Drawing for the job (mm, zero at the part's lowest x, y, z). A direction names the side the tool comes from. Give positions to 0.01 mm unless a question says otherwise; leave off trailing zeros. Loops run counter-clockwise (first coordinate to the right, second up) from the corner with the lowest first, then second, coordinate; pieces in that order, holes last. Notation, with made-up numbers: M 54,0 L 86,0 A4 ccw 86,4 Z; hole C -34.5,3 d5. An arc over 180 degrees is marked long. Answer in a Markdown table with one row per item. Add a question column.
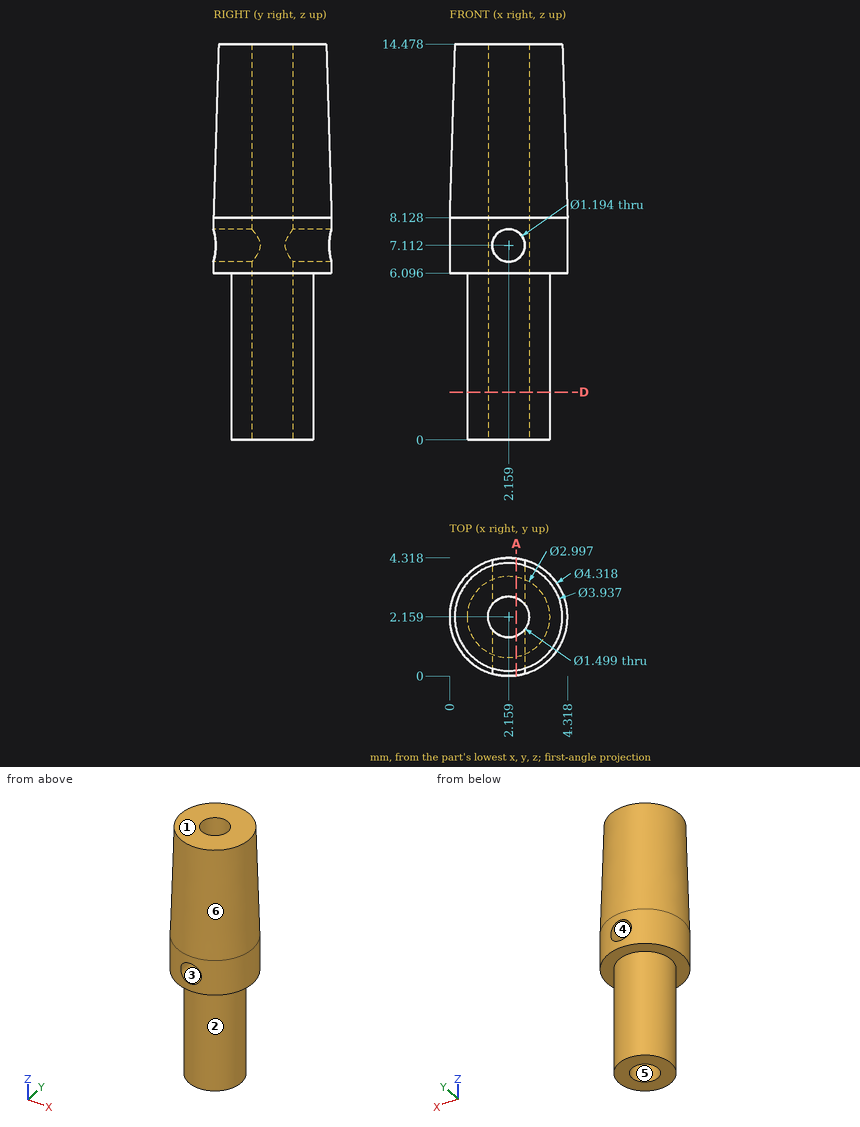
(1) Pin check, flat tip, straight feed: pin 1 (1.5 mm diameter, centred on y = 3.5, z = 2.5, fed in from -X). Stop position of the tip, or through.
(2) Wall check: line 1 (Y direction, x = 2.3, z = 7.75) (1 decimal); line 2 (Z direction, x = 0.95, y = 1.05); line 3 (Z direction, x = 1.7, y = 3.8) (1 decimal). Give the ranges that are in metal, low to high.
(3) Slice it at A-A, the plane x = 2.45. State how many separate pieces and enclosed holes the cut face has.
(4) Slice it at D-D, the plane z = 1.75. Give the cut face in (x, y).
(5) Pull direction Z, two halves, no side cores. Call the marked faces 3, 4, 5 and 6: +Z half, -Z half, draft (parallel to the pull), parting line (faces both ways), or undercut.
(6) Tool access for the marked faces 1 and 2: list every direction of +Z, -Z, +X, -X, +Y, -Y with a clear straight run to the whole face (end or side of a thin tool).
Solution:
| question | item | result |
|---|---|---|
| 1 | pin 1 | x = 0.78 |
| 2 | line 1 | 0 to 1.4, 2.9 to 4.3 |
| 2 | line 2 | 6.1 to 14.48 |
| 2 | line 3 | 6.1 to 6.7, 7.5 to 14.5 |
| 3 | separate pieces | 4 |
| 3 | enclosed holes | 0 |
| 4 | outline | C 2.16,2.16 d3; hole C 2.16,2.16 d1.5 |
| 5 | face 3 | undercut |
| 5 | face 4 | undercut |
| 5 | face 5 | draft |
| 5 | face 6 | +Z half |
| 6 | face 1 | +Z, +X, -X, +Y, -Y |
| 6 | face 2 | -Z |
